Geometry: see drawing. Coordinates: mm, zero at the bounding-box minimum. A direction names the side the tool comes from. Coordinates: 2 decimals unless noted, no trailing zeros. Order: outer loops, then holes, each group sorted by start corner. A loop starts at its lowest first (then second) coordinate and runs counter-clockwise, first axis right, second up.
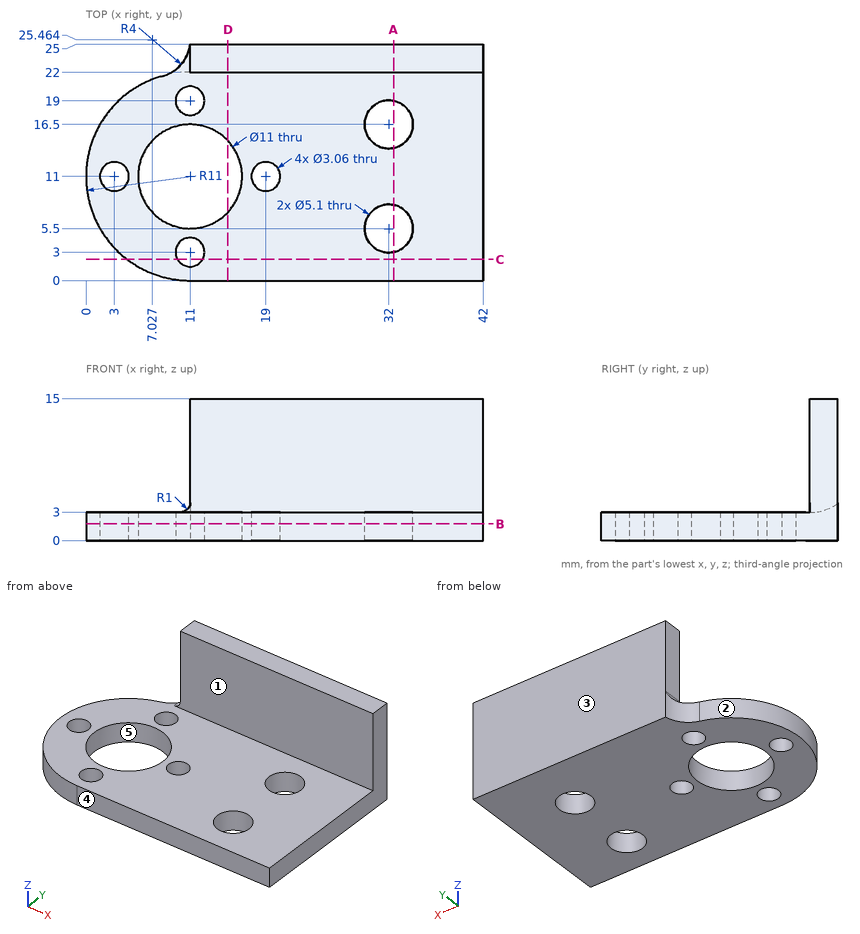
Q1. Set-up query: the marked faces 1 and 2. Return all of +Z, -Z, +X, -X, +Y, -Y with unobstructed straight access to the full face (end or side cutting, diameter ignored); none if empty.
Solutions:
face 1: +Z, +X, -X, -Y
face 2: +Z, -Z, -X
Q2. Section query C-C on y = 2.25. Output: boundary loops of the cut face in (x, z), plus the area to 3 significant figures.
Solutions:
outline: (4.33, 0) - (9.67, 0) - (9.67, 3) - (4.33, 3) - close; (12.33, 0) - (42, 0) - (42, 3) - (12.33, 3) - close
area: 105 mm2
Q3. Material intervals for line 1 along Y through (x, z) = (32, 0.85); line 2 along Z through (x, y) = (26.5, 18); line 3 along Y through (x, z) = (19, 1.8), sorted ascending.
Solutions:
line 1: y = 0 to 2.95, 8.05 to 13.95, 19.05 to 25
line 2: z = 0 to 3
line 3: y = 0 to 9.47, 12.53 to 25
Q4. Section query D-D on x = 15. Output: boundary loops of the cut face in (y, z) (1 decimal).
Solutions:
outline: (0, 0) - (7.2, 0) - (7.2, 3) - (0, 3) - close; (14.8, 0) - (25, 0) - (25, 15) - (22, 15) - (22, 3) - (14.8, 3) - close
Q5. Section query B-B on z = 1.75. Output: boundary loops of the cut face in (x, y), plus the area to 3 significant figures.
Solutions:
outline: (8.09, 21.61) arc R11 ccw to (11, 0) - (42, 0) - (42, 25) - (11, 25) arc R4 cw to start; hole circle Ø3.06 at (3, 11); hole circle Ø11 at (11, 11); hole circle Ø3.06 at (11, 3); hole circle Ø3.06 at (11, 19); hole circle Ø3.06 at (19, 11); hole circle Ø5.1 at (32, 5.5); hole circle Ø5.1 at (32, 16.5)
area: 802 mm2
Q6. Pin query (flat end, axial travel): P1, Ø6, axis at x = 33, y = 3, coming from the +Z side; P2, Ø1.5, axis at x = 12, z = 8.5, coming from the -Y side; P3, Ø2, axis at x = 8.5, z = 3.5, coming from the -Y side; P4, Ø4, axis at x = 19, y = 11, coming from the -Z side. Return the tip coordinate at first contact, or that it passes through.
Solutions:
P1: stops at z = 3
P2: stops at y = 22
P3: stops at y = 0.12
P4: stops at z = 0
Q7. Section query A-A on x = 32.5. Output: boundary loops of the cut face in (y, z).
Solutions:
outline: (0, 0) - (3, 0) - (3, 3) - (0, 3) - close; (8, 0) - (14, 0) - (14, 3) - (8, 3) - close; (19, 0) - (25, 0) - (25, 15) - (22, 15) - (22, 3) - (19, 3) - close
Q8. Pull-direction query (Y, two-part tool) for the marked faces 3, 4 and 5; classes: pulls with the +Y half, pulls with the -Y half, needs draft (parallel to the pull), parting line crosses it, or undercut.
Solutions:
face 3: pulls with the +Y half
face 4: pulls with the -Y half
face 5: undercut
